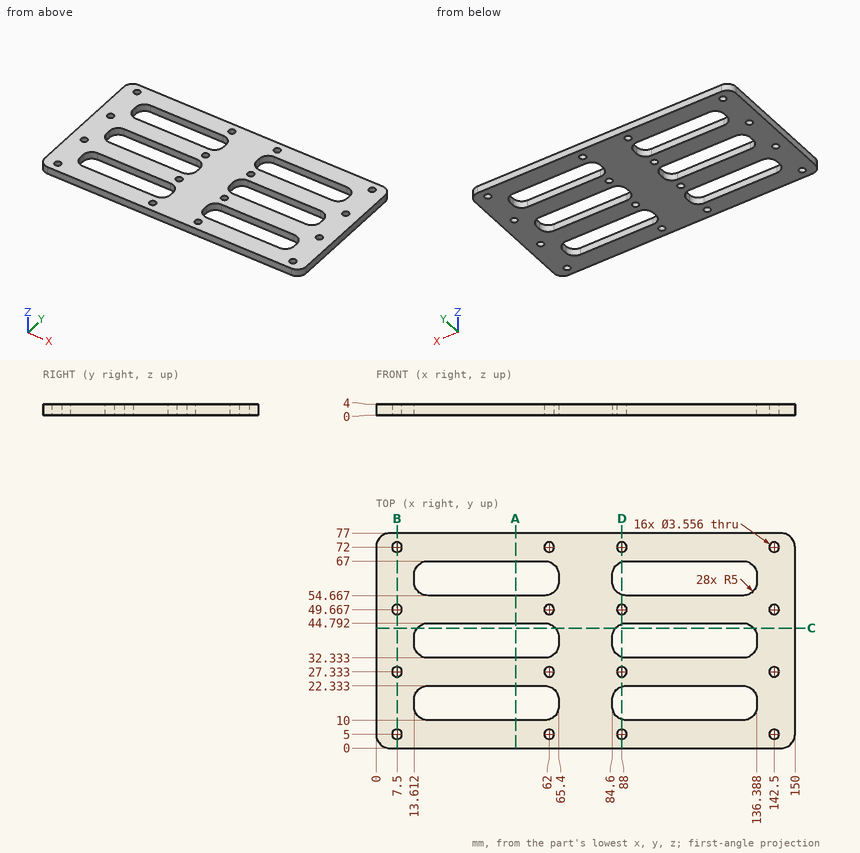
Could you check a few things on this drawing? It's one solid part, dimensions in mm from its lowest x, y, z. Coordinates: 2 decimals unless noted, no trailing zeros. Loops run counter-clockwise (first coordinate to the right, second up) from the corner with the lowest first, then second, coordinate; pieces in that order, holes last.
1. Imagine slicing it at A-A (x = 50). Please give me the cut outline in (y, z).
2. Imagine slicing it at D-D (x = 88). Give the number of separate pieces and of enclosed holes in the cut face, and give its area (3 significant figures).
3. Imagine slicing it at B-B (x = 7.5). Please give me the cut outline in (y, z) (1 decimal), and give its area (3 significant figures).
4. I need wall thicknesses on L1, parallel to Y at x = 125.5, z = 1.35; L2, parallel to X at y = 61, z = 2.55; L3, parallel to Y at x = 7.5, z = 2.5 (1 decimal). Which ranges of each line are inside material? Lowest first, please.
5. Imagine slicing it at C-C (y = 43). Please give me the cut outline in (x, z) (1 decimal).
Computed values:
1. outline: (0, 0) - (10, 0) - (10, 4) - (0, 4) - close; (22.33, 0) - (32.33, 0) - (32.33, 4) - (22.33, 4) - close; (44.79, 0) - (54.67, 0) - (54.67, 4) - (44.79, 4) - close; (67, 0) - (77, 0) - (77, 4) - (67, 4) - close
2. separate pieces: 8
2. enclosed holes: 0
2. area: 109 mm2
3. outline: (0, 0) - (3.2, 0) - (3.2, 4) - (0, 4) - close; (6.8, 0) - (25.6, 0) - (25.6, 4) - (6.8, 4) - close; (29.1, 0) - (47.9, 0) - (47.9, 4) - (29.1, 4) - close; (51.4, 0) - (70.2, 0) - (70.2, 4) - (51.4, 4) - close; (73.8, 0) - (77, 0) - (77, 4) - (73.8, 4) - close
3. area: 251 mm2
4. L1: y = 0 to 10, 22.33 to 32.33, 44.79 to 54.67, 67 to 77
4. L2: x = 0 to 13.61, 65.4 to 84.6, 136.39 to 150
4. L3: y = 0 to 3.2, 6.8 to 25.6, 29.1 to 47.9, 51.4 to 70.2, 73.8 to 77
5. outline: (0, 0) - (14.8, 0) - (14.8, 4) - (0, 4) - close; (64.2, 0) - (85.8, 0) - (85.8, 4) - (64.2, 4) - close; (135.2, 0) - (150, 0) - (150, 4) - (135.2, 4) - close
